Read the model definition and answer for the solid it produces. Units are mm, in the model's axes. A direction names the side the tool comes from. Give positions to 0.01 mm unless a question says otherwise; leave off trailing zeros. Loops run counter-clockwise (first coordinate to the right, second up) from the corner with the lowest first, then second, coordinate; pieces in that order, holes last. Notation, with made-up numbers: M 14.25,0.5 L 23.25,0.5 A20 cw 23.25,21.5 Z; hole C 9.5,14.25 d3. An arc over 180 degrees is marked long. Return JSON: item names as keys, results as strings. Group by question number.
```python
from build123d import *

# Parameters (mm, degrees)
SKETCH_1_W      = 53.34
SKETCH_1_H      = 68.58
SKETCH_1_R      = 1.585
EXTRUDE_1_DEPTH = 1.5
SKETCH_2_R      = 3.25
EXTRUDE_2_DEPTH = 8
SKETCH_3_W      = 12
SKETCH_3_H      = 5.3
EXTRUDE_3_DEPTH = 6
SKETCH_4_W      = 2.8
SKETCH_4_H      = 4
EXTRUDE_4_DEPTH = 2
SKETCH_5_W      = 4.8
SKETCH_5_H      = 44
EXTRUDE_5_DEPTH = 4
SKETCH_6_W      = 9
SKETCH_6_H      = 8
EXTRUDE_6_DEPTH = 3


with BuildPart() as part:
    # 草图1 → 凸台-拉伸1 (new body)
    with BuildSketch(Plane.XY):
        with Locations((26.67, 34.29)):
            Rectangle(SKETCH_1_W, SKETCH_1_H)
        with Locations((48.92, 64.16)):
            Circle(SKETCH_1_R, mode=Mode.SUBTRACT)
        with Locations((4.42, 64.16)):
            Circle(SKETCH_1_R, mode=Mode.SUBTRACT)
        with Locations((4.42, 4.42)):
            Circle(SKETCH_1_R, mode=Mode.SUBTRACT)
        with Locations((48.92, 4.42)):
            Circle(SKETCH_1_R, mode=Mode.SUBTRACT)
    extrude(amount=EXTRUDE_1_DEPTH)

    # 草图2 → 凸台-拉伸2 (add)
    with BuildSketch(Plane.XY.offset(1.5)):
        with Locations(Location((38.82, 58.16, 0), (0, 0, 180))):
            Circle(SKETCH_2_R)
    extrude(amount=EXTRUDE_2_DEPTH)

    # 草图3 → 凸台-拉伸3 (add)
    with BuildSketch(Plane.XY.offset(1.5)):
        with Locations((32.52, 46.11)):
            Rectangle(SKETCH_3_W, SKETCH_3_H)
    extrude(amount=EXTRUDE_3_DEPTH)

    # 草图4 → 凸台-拉伸4 (add)
    with BuildSketch(Plane.XY.offset(1.5)):
        with Locations((34.44, 11.3)):
            Rectangle(SKETCH_4_W, SKETCH_4_H)
    extrude(amount=EXTRUDE_4_DEPTH)

    # 草图5 → 凸台-拉伸5 (add)
    with BuildSketch(Plane(origin=(0, 0, 0), x_dir=(-1, 0, 0), z_dir=(0, 0, -1))):
        with Locations((-49.04, 34.4)):
            Rectangle(SKETCH_5_W, SKETCH_5_H)
        with Locations((-4.3, 34.4)):
            Rectangle(SKETCH_5_W, SKETCH_5_H)
    extrude(amount=EXTRUDE_5_DEPTH)

    # 草图6 → 凸台-拉伸6 (add)
    with BuildSketch(Plane.XY.offset(1.5)):
        with Locations((40.44, 4)):
            Rectangle(SKETCH_6_W, SKETCH_6_H)
    extrude(amount=EXTRUDE_6_DEPTH)


solid = part.part
```
1. Flat-ended cylindrical pins translate along their axes: P1, Ø6, axis at x = 10.5, y = 9, coming from the +Z side; P2, Ø1, axis at y = 12, z = 3, coming from the +X side; P3, Ø2.5, axis at y = 2.5, z = 3, coming from the +X side; P4, Ø6.5, axis at x = 31.5, z = 4, coming from the +Y side. Find the tip coordinate at first contact, or state that the pin passes through.
2. The mould has two halves that part along X. Classify faces 1 (the flat face through (26, 35, 0)), 2 (the flat face through (26, 68.58, 1)), 3 (the flat face through (38.52, 46, 4)): +X half, -X half, draft (parallel to the pull), parting line (faces both ways), or undercut.
3. Find section D-D (z = 5.5). Write down the section's boundary in (x, y), and give its area (3 significant figures).
4. Straight lines are drawn through the part: line 1 along Y through (x, z) = (4.42, 1.1) (3 decimals); line 2 along X through (y, z) = (64.16, 0.5) (3 decimals); line 3 along X through (y, z) = (33, -2). For each, find the intervals that lie inside material, in ascending order.
5. For faces 4 (the flat face through (46.64, 34, -2)), 5 (the flat face through (4, 12.4, -2)), 6 (the flat face through (51.44, 34, -2)), 7 (the flat face through (32, 46, 7.5)), determine the directions among +Z, -Z, +X, -X, +Y, -Y from which every point of the face is accessible in a straight line to the end or side of a thin tool.
6. Find section A-A (y = 64.16). Write down the section's boundary in (x, z) (3 decimals).
7. Find section C-C (y = 41). Write down the section's boundary in (x, z), and give its area (3 significant figures).
8. Find section B-B (x = 4.42). Write down the section's boundary in (y, z) (3 decimals).
Result:
{
 "1": {"P1": "stops at z = 1.5", "P2": "stops at x = 35.84", "P3": "stops at x = 44.94", "P4": "stops at y = 68.58"},
 "2": {"face 1": "undercut", "face 2": "draft", "face 3": "+X half"},
 "3": {"outline": "M 26.52,43.46 L 38.52,43.46 L 38.52,48.76 L 26.52,48.76 Z; C 38.82,58.16 d6.5", "area": "96.8 mm2"},
 "4": {"line 1": "y = 0 to 2.835, 6.005 to 62.575, 65.745 to 68.58", "line 2": "x = 0 to 2.835, 6.005 to 47.335, 50.505 to 53.34", "line 3": "x = 1.9 to 6.7, 46.64 to 51.44"},
 "5": {"face 4": "-Z, +Y, -Y", "face 5": "-Z, +X, -X, -Y", "face 6": "-Z, +X, +Y, -Y", "face 7": "+Z, +X, -X, -Y"},
 "6": {"outline": "M 0,0 L 2.835,0 L 2.835,1.5 L 0,1.5 Z; M 6.005,0 L 47.335,0 L 47.335,1.5 L 6.005,1.5 Z; M 50.505,0 L 53.34,0 L 53.34,1.5 L 50.505,1.5 Z"},
 "7": {"outline": "M 0,0 L 1.9,0 L 1.9,-4 L 6.7,-4 L 6.7,0 L 46.64,0 L 46.64,-4 L 51.44,-4 L 51.44,0 L 53.34,0 L 53.34,1.5 L 0,1.5 Z", "area": "118 mm2"},
 "8": {"outline": "M 0,0 L 2.835,0 L 2.835,1.5 L 0,1.5 Z; M 6.005,0 L 12.4,0 L 12.4,-4 L 56.4,-4 L 56.4,0 L 62.575,0 L 62.575,1.5 L 6.005,1.5 Z; M 65.745,0 L 68.58,0 L 68.58,1.5 L 65.745,1.5 Z"}
}
